For this review, take the finished solid that the model builds, in its own axes (mm). Face numbers are marked on the shaded views. Coordinates: 2 decimals unless noted, no trailing zeros. Write each loop counter-clockwise with the first axis right and the second up, starting at its lowest first coordinate (ties: lowest second). Pieces come first, ordered by that corner, then holes. Notation, with made-up numbers: M -16.75,64 L 7.25,64 A22 cw 7.25,87 Z; hole C 15.5,-35.5 d2. An arc over 180 degrees is marked long. Return JSON: item names as keys, results as strings.
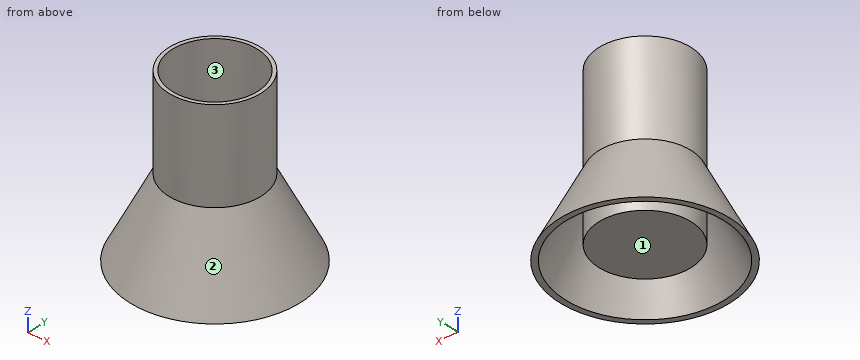
```python
from build123d import *

# Parameters (mm, degrees)
F0_R        = 32.5
F0_R_2      = 30
F1_DEPTH    = 120
F1_FACE_R   = 32.5
F1_FACE_R_2 = 30
F4_DEPTH    = 10
F5_DEPTH    = 14
F5_FACE_R   = 30
F6_DEPTH    = 10


with BuildPart() as f1:
    # F0 (on Top) → F1 (new body)
    with BuildSketch(Plane.XY):
        Circle(F0_R)
        Circle(F0_R_2, mode=Mode.SUBTRACT)
    extrude(amount=F1_DEPTH)

    # F2 (on Right) → F3 (revolve)
    with BuildSketch(Plane.YZ):
        Polygon((-56, 0), (-30, 52), (-30, 60), (-60, 0), align=None)
    revolve(axis=Axis((0, 0, 30), (0, 0, 1)))

    # F1_face (on face) → F4 (cut)
    with BuildSketch(Plane(origin=(0, 0, 0), x_dir=(1, 0, 0), z_dir=(0, 0, -1))):
        Circle(F1_FACE_R)
        Circle(F1_FACE_R_2, mode=Mode.SUBTRACT)
    extrude(amount=-F4_DEPTH, mode=Mode.SUBTRACT)

    # F0 (on Top) → F5 (join)
    with BuildSketch(Plane.XY):
        Circle(F0_R_2)
    extrude(amount=F5_DEPTH)

    # F5_face (on face) → F6 (cut)
    with BuildSketch(Plane(origin=(0, 0, 0), x_dir=(1, 0, 0), z_dir=(0, 0, -1))):
        Circle(F5_FACE_R)
    extrude(amount=-F6_DEPTH, mode=Mode.SUBTRACT)


solid = f1.part
```
1. We need section B-B (y = 0). State the section outline as (x, z) points, plus the area to 3 significant figures.
Checks:
{"outline": "M -60,0 L -56,0 L -32.5,47 L -32.5,10 L 32.5,10 L 32.5,47 L 56,0 L 60,0 L 32.5,55 L 32.5,120 L 30,120 L 30,14 L -30,14 L -30,120 L -32.5,120 L -32.5,55 Z", "area": "1,200 mm2"}
2. We need section C-C (z = 52). State the section outline as (x, y) points, plus the area to 3 significant figures.
Checks:
{"outline": "C 0,0 d68; hole C 0,0 d60", "area": "804 mm2"}
3. Wall thickness on L1, parallel to Y at x = -16, z = 35; L2, parallel to Y at x = 0, z = 36; L3, parallel to X at y = 20.5, z = 16: over which ranges is each line inside the solid? List them lowest first. Write a range as from..to.
Checks:
{"L1": "-39.37..-35.02, -28.29..-25.38, 25.38..28.29, 35.02..39.37", "L2": "-42..-38, -32.5..-30, 30..32.5, 38..42", "L3": "-47.79..-43.4, -25.22..-21.9, 21.9..25.22, 43.4..47.79"}
4. Clearance check with flat-ended pins moving along their axes: pin 1 Ø1.5 at (x, y) = (3.5, -34.5) entering from -Z; pin 2 Ø5 at (x, z) = (-7, 105) entering from +Y; pin 3 Ø4 at (y, z) = (13, 101) entering from +X. State where each tip first meets the part, or that it passes through.
Checks:
{"pin 1": "z = 41.15", "pin 2": "y = 32.19", "pin 3": "x = 30.58"}
5. Draft analysis for pull direction Y (two halves, no side actions). For the marked faces 1, 2 and 3, state which applies: +Y half, -Y half, draft (parallel to the pull), parting line (faces both ways), or undercut.
Checks:
{"face 1": "undercut", "face 2": "parting line", "face 3": "undercut"}
6. We need section A-A (z = 27.5). State the section outline as (x, y) points, plus the area to 3 significant figures.
Checks:
{"outline": "C 0,0 d92.5; C 0,0 d65; hole C 0,0 d84.5; hole C 0,0 d60", "area": "1,600 mm2"}
